```python
from build123d import *

# Parameters (mm, degrees)
SKETCH1_R           = 50
SKETCH1_R_2         = 5
BOSS_EXTRUDE1_DEPTH = 6
SKETCH2_R           = 2.5
CUT_EXTRUDE1_DEPTH  = 7


with BuildPart() as part:
    # Sketch1 → Boss-Extrude1 (new body)
    with BuildSketch(Plane.XY):
        Circle(SKETCH1_R)
        Circle(SKETCH1_R_2, mode=Mode.SUBTRACT)
    extrude(amount=BOSS_EXTRUDE1_DEPTH)

    # Sketch2 → Cut-Extrude1 (cut, through all)
    with BuildSketch(Plane(origin=(0, 0, 0), x_dir=(-1, 0, 0), z_dir=(0, 0, -1))):
        with Locations((0, 20)):
            Circle(SKETCH2_R)
        with Locations((20, 0)):
            Circle(SKETCH2_R)
        with Locations((0, -20)):
            Circle(SKETCH2_R)
        with Locations((-20, 0)):
            Circle(SKETCH2_R)
    extrude(amount=-CUT_EXTRUDE1_DEPTH, mode=Mode.SUBTRACT)


solid = part.part
```
Check sheet for the modelled part. Datum: model origin and axes. Units: mm. Give positions to 0.01 mm unless a question says otherwise; leave off trailing zeros. Loops run counter-clockwise (first coordinate to the right, second up) from the corner with the lowest first, then second, coordinate; pieces in that order, holes last. Notation, with made-up numbers: M 8.5,70 L 54.5,70 A18 ccw 54.5,92 Z; hole C 60.5,31 d9. An arc over 180 degrees is marked long. Answer in a Markdown table with one row per item.
1) Cross-section at A-A (x = 0). Enter the section's corners in (y, z).
Solutions:
| item | result |
|---|---|
| outline | M -50,0 L -22.5,0 L -22.5,6 L -50,6 Z; M -17.5,0 L -5,0 L -5,6 L -17.5,6 Z; M 5,0 L 17.5,0 L 17.5,6 L 5,6 Z; M 22.5,0 L 50,0 L 50,6 L 22.5,6 Z |
2) Mould release check, pull along Y, two halves, no side actions. Record for faces 1 (the face through (-1, -10, 0)), 2 (the face through (47.69, 15.02, 2.96)), 3 (the face through (-17.5, 0.1, 3)): released by +Y, released by -Y, zero draft, split by the parting line, or undercut.
Solutions:
| item | result |
|---|---|
| face 1 | zero draft |
| face 2 | split by the parting line |
| face 3 | undercut |
3) Cross-section at C-C (z = 0.95). Enter the section's corners in (x, y), plus the area to 3 significant figures.
Solutions:
| item | result |
|---|---|
| outline | C 0,0 d100; hole C -20,0 d5; hole C 0,0 d10; hole C 0,-20 d5; hole C 0,20 d5; hole C 20,0 d5 |
| area | 7,700 mm^2 |
4) Thickness scan on line 1 (Y direction, x = 0, z = 4.75); line 2 (Y direction, x = -19.5, z = 4.7); line 3 (X direction, y = -22, z = 4.35). Record the ranges inside material, lowest first.
Solutions:
| item | result |
|---|---|
| line 1 | y = -50 to -22.5, -17.5 to -5, 5 to 17.5, 22.5 to 50 |
| line 2 | y = -46.04 to -2.45, 2.45 to 46.04 |
| line 3 | x = -44.9 to -1.5, 1.5 to 44.9 |
5) Depth check by flat-ended pin: pin 1 (1.5 mm diameter, centred on x = -34, z = 4.5, fed in from -Y); pin 2 (8 mm diameter, centred on x = -20, y = 0, fed in from -Z); pin 3 (3 mm diameter, centred on x = 17.5, z = 1.5, fed in from +Y). Enter the tip coordinate at first touch or a pass-through.
Solutions:
| item | result |
|---|---|
| pin 1 | stops at y = -37.34 |
| pin 2 | stops at z = 0 |
| pin 3 | stops at y = 47.37 |
6) Cross-section at D-D (y = -20). Enter the section's corners in (x, z), plus the area to 3 significant figures.
Solutions:
| item | result |
|---|---|
| outline | M -45.83,0 L -2.5,0 L -2.5,6 L -45.83,6 Z; M 2.5,0 L 45.83,0 L 45.83,6 L 2.5,6 Z |
| area | 520 mm^2 |
